from build123d import *

# Parameters (mm, degrees)
EXTRU_MINCE2_DEPTH      = 100
ENL_V_MAT_EXTRU_2_DEPTH = 100


with BuildPart() as part:
    # Esquisse3 → Extru.-Mince2 (new body)
    with BuildSketch(Plane.XY):
        with BuildLine():
            ThreePointArc((15.315208394, 15.793808656), (20.193436478, 8.730700042), (21.997396912, 0.338421491))
            ThreePointArc((21.997396912, 0.338421491), (0.169215751, -21.999349218), (-22, 0))
            ThreePointArc((-22, 0), (-20.325349715, 8.419035512), (-15.556349186, 15.556349186))
            Line((-15.556349186, 15.556349186), (-19.798989873, 19.798989873))
            ThreePointArc((-19.798989873, 19.798989873), (-25.86862691, 10.715136106), (-28, 0))
            ThreePointArc((-28, 0), (0.215365501, -27.999171732), (27.996686979, 0.430718261))
            ThreePointArc((27.996686979, 0.430718261), (25.700737335, 11.111800054), (19.49208341, 20.101211017))
            Line((19.49208341, 20.101211017), (15.315208394, 15.793808656))
        make_face()
    extrude(amount=EXTRU_MINCE2_DEPTH)

    # Esquisse7 → Enlèv. mat.-Extru.2 (cut)
    with BuildSketch(Plane.XY.offset(100)):
        with BuildLine():
            Line((-26, 0), (-24, 0))
            ThreePointArc((-24, 0), (0, 24), (24, 0))
            Line((24, 0), (26, 0))
            ThreePointArc((26, 0), (0, 26), (-26, 0))
        make_face()
    extrude(amount=-ENL_V_MAT_EXTRU_2_DEPTH, mode=Mode.SUBTRACT)


solid = part.part
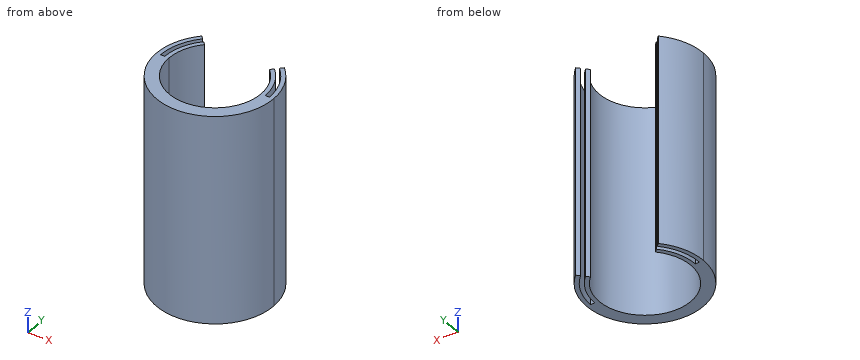
Could you check a few things on this model? Use its own coordinates, in mm. Give positions to 0.01 mm unless a question says otherwise; leave off trailing zeros. Order: outer loops, then holes, each group sorted by start corner. A loop starts at its lowest first (then second) coordinate and runs counter-clockwise, first axis right, second up. Notation, with made-up numbers: (87.25, 87.5) -> (99.25, 87.5) arc R4 cw to (99.25, 93.5) -> close; hole circle Ø3 at (64, 60). An arc over 180 degrees is marked (long way). Answer in a Markdown table with one row per item. Add a question column.
Item 1: Imagine slicing it at D-D (x = 0). List the corners of the cut face in (y, z) for me, and give its area (3 significant figures).
Item 2: Imagine slicing it at B-B (y = -9.5). List the corners of the cut face in (x, z) for me, and give its area (3 significant figures).
Item 3: I'm going to push flat-ended pins straight in: P1, Ø10, axis at y = -19, z = 60.5, coming from the -X side; P2, Ø3, axis at y = -2.5, z = 78.5, coming from the -X side; P3, Ø3, axis at x = 18, z = 18.5, coming from the -Y side. Where does each tip first touch, or does it pass through?
Item 4: Imagine slicing it at C-C (x = -23). List the corners of the cut face in (y, z) for me.
Item 5: Imagine slicing it at A-A (z = 43). List the corners of the cut face in (x, y) for me.
Item 6: Please list where these lines run through material, in increasing order: probe 1 along X at (y, z) = (6.5, 66); probe 2 along Y at (x, z) = (0, 33); probe 3 along X at (y, z) = (-1.5, 51).
Result:
| question | item | result |
|---|---|---|
| 1 | outline | (-28, 0) -> (-22, 0) -> (-22, 100) -> (-28, 100) -> close |
| 1 | area | 600 mm2 |
| 2 | outline | (-26.34, 0) -> (-19.84, 0) -> (-19.84, 100) -> (-26.34, 100) -> close; (19.84, 0) -> (26.34, 0) -> (26.34, 100) -> (19.84, 100) -> close |
| 2 | area | 1,300 mm2 |
| 3 | P1 | x = -24.25 |
| 3 | P2 | x = -27.98 |
| 3 | P3 | y = -22.62 |
| 4 | outline | (-15.97, 0) -> (6.86, 0) -> (6.86, 100) -> (-15.97, 100) -> close; (12.12, 0) -> (15.97, 0) -> (15.97, 100) -> (12.12, 100) -> close |
| 5 | outline | (-26, 0) arc R26 cw to (-18.38, 18.38) -> (-19.8, 19.8) arc R28 ccw (long way) to (19.49, 20.1) -> (18.1, 18.67) arc R26 cw to (26, 0) -> (24, 0) arc R24 ccw to (16.71, 17.23) -> (15.32, 15.79) arc R22 cw (long way) to (-15.56, 15.56) -> (-16.97, 16.97) arc R24 ccw to (-24, 0) -> close |
| 6 | probe 1 | -27.24 to -25.17, -23.1 to -21.02, 21.02 to 23.1, 25.17 to 27.24 |
| 6 | probe 2 | -28 to -22 |
| 6 | probe 3 | -27.96 to -21.95, 21.95 to 27.96 |
